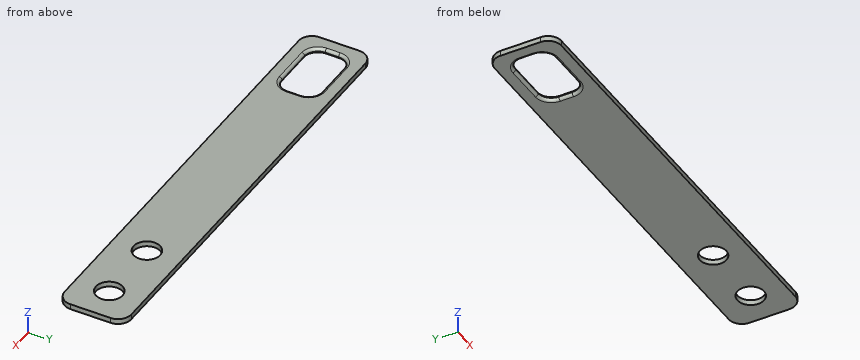
Autodesk Inventor part; units mm, degrees
ref_plane "YZ Plane" through (0, 0, 0) normal (1, 0, 0) x (0, 1, 0)
ref_plane "XZ Plane" through (0, 0, 0) normal (0, 1, 0) x (-1, 0, 0)
ref_plane "XY Plane" through (0, 0, 0) normal (0, 0, 1) x (1, 0, 0)
ref_plane "Arbeitsebene1" through (0, 0, 0) normal (0, 0, 1) x (1, 0, 0)
sketch "Skizze1" plane through (0, 0, 0) normal (0, 0, 1) x (1, 0, 0)
  circle A0 centre (118, -9.35) radius 5 construction
  circle A1 centre (118, -9.35) radius 5
  circle A2 centre (93, -9.35) radius 5 construction
  circle A3 centre (93, -9.35) radius 5
  line L0 (130.5, -21.85) -> (-35, -21.85)
  line L1 (-35, -21.85) -> (-35, 3.15)
  line L2 (-35, 3.15) -> (130.5, 3.15)
  line L3 (130.5, 3.15) -> (130.5, -21.85)
  line L4 (-30, -16.85) -> (-5, -16.85)
  line L5 (-5, -16.85) -> (-5, -1.85)
  line L6 (-5, -1.85) -> (-30, -1.85)
  line L7 (-30, -1.85) -> (-30, -16.85)
  line L8 (0, -2.2) -> (0, -28) construction
  point P0 (0, 0)
  dimension "d0" = 12.5
  dimension "d1" = 25
  dimension "d2" = 12.5
  dimension "d3" = 5
  dimension "d4" = 5
  dimension "d5" = 5
  dimension "d6" = 25
  dimension "d7" = 5
  dimension "d8" = 15
extrude "Extrusion1" add sketch "Skizze1" along normal blind 2
fillet "Rundung1" radius 5 8 edges at (-5, -16.85, 1) (-30, -16.85, 1) (-30, -1.85, 1) (-5, -1.85, 1) (-35, -21.85, 1) (-35, 3.15, 1) (130.5, -21.85, 1) (130.5, 3.15, 1)
fillet "Rundung2" radius 1 16 edges at (-17.5, -1.85, 2) (-28.5355, -3.3145, 2) (-30, -9.35, 2) (-28.5355, -15.3855, 2) (-17.5, -16.85, 2) (-6.4645, -15.3855, 2) (-5, -9.35, 2) (-6.4645, -3.3145, 2) (-5, -9.35, 0) (-6.4645, -15.3855, 0) (-17.5, -16.85, 0) (-28.5355, -15.3855, 0) (-30, -9.35, 0) (-28.5355, -3.3145, 0) (-17.5, -1.85, 0) (-6.4645, -3.3145, 0)
equation "\"d1\" = 2 * d0"
equation "\"d2\" = d0"
equation "\"d4\" = d3"
equation "\"d5\" = d3"
equation "\"d7\" = d3"
properties part number "hangmount"
Build history of the part. All positions in model axes, mm. Round coordinates to 2 decimals unless told otherwise and drop trailing zeros. Write each loop counter-clockwise with the first axis right and the second up, starting at its lowest first coordinate (ties: lowest second). Pieces come first, ordered by that corner, then holes. Notation, with made-up numbers: (-19, 58) -> (-10, 58) arc R23 cw to (-10, 92) -> close; hole circle Ø4 at (-34.5, 79.5). An arc over 180 degrees is marked (long way). Write item = value, one per line.
(1) Band-saw the part on C-C (z = 0.5). Give the cut face in (x, y).
Answer:
outline = (-35, -16.85) arc R5 ccw to (-30, -21.85) -> (125.5, -21.85) arc R5 ccw to (130.5, -16.85) -> (130.5, -1.85) arc R5 ccw to (125.5, 3.15) -> (-30, 3.15) arc R5 ccw to (-35, -1.85) -> close; hole (-30.13, -11.85) arc R5.13 ccw to (-25, -16.98) -> (-10, -16.98) arc R5.13 ccw to (-4.87, -11.85) -> (-4.87, -6.85) arc R5.13 ccw to (-10, -1.72) -> (-25, -1.72) arc R5.13 ccw to (-30.13, -6.85) -> close; hole circle Ø10 at (93, -9.35); hole circle Ø10 at (118, -9.35)
(2) Band-saw the part on B-B (x = 93). Give the cut face in (y, z).
Answer:
outline = (-21.85, 0) -> (-14.35, 0) -> (-14.35, 2) -> (-21.85, 2) -> close; (-4.35, 0) -> (3.15, 0) -> (3.15, 2) -> (-4.35, 2) -> close
(3) Probe L1, parallel to Y at x = 118, z = 1.05; L2, parallel to X at y = -12.5, z = 0.3; L3, parallel to X at y = -10, z = 1.4. List the from-to ranges inside material, lowest first.
Answer:
L1 = -21.85 to -14.35, -4.35 to 3.15
L2 = -35 to -30.25, -4.75 to 89.12, 96.88 to 114.12, 121.88 to 130.5
L3 = -35 to -30.08, -4.92 to 88.04, 97.96 to 113.04, 122.96 to 130.5
(4) Flat gauge pin, fed straight in: pin 1 (11.5 mm diameter, centred on x = 93, y = -9.35, fed in from -Z). Where does the tip first touch, or does it go through?
Answer:
pin_1 = 0
(5) Band-saw the part on A-A (y = -9.35). State how many separate pieces and enclosed holes the cut face has, then the cut area to 3 significant figures.
Answer:
separate_pieces = 4
enclosed_holes = 0
area = 240 mm2
